```python
from build123d import *

# Parameters (mm, degrees)
SKETCH1_R           = 25
BOSS_EXTRUDE1_DEPTH = 2
SKETCH2_R           = 15
CUT_EXTRUDE1_DEPTH  = 5
CUT_EXTRUDE4_DEPTH  = 10
CIRPATTERN3_COUNT   = 20
CUT_EXTRUDE5_DEPTH  = 10
CIRPATTERN4_COUNT   = 10


with BuildPart() as part:
    # Sketch1 → Boss-Extrude1 (new body)
    with BuildSketch(Plane.XY):
        Circle(SKETCH1_R)
    extrude(amount=BOSS_EXTRUDE1_DEPTH)

    # Sketch2 → Cut-Extrude1 (cut)
    with BuildSketch(Plane(origin=(0, 0, 0), x_dir=(-1, 0, 0), z_dir=(0, 0, -1))):
        Circle(SKETCH2_R)
    extrude(amount=-CUT_EXTRUDE1_DEPTH, mode=Mode.SUBTRACT)

    # Sketch8 → Cut-Extrude4 (cut)
    with BuildSketch(Plane.XY.offset(2)):
        with BuildLine():
            Line((-1.502861851, 23.143578335), (-1.0312505, 16.38824879))
            Line((-1.0312505, 16.38824879), (1.0312505, 16.38824879))
            Line((1.0312505, 16.38824879), (1.478722794, 23.143578335))
            ThreePointArc((1.478722794, 23.143578335), (-0.012069528, 24.634370658), (-1.502861851, 23.143578335))
        make_face()
    cut_extrude4 = extrude(amount=-CUT_EXTRUDE4_DEPTH, mode=Mode.SUBTRACT)

    # CirPattern3: Cut-Extrude4 ×20 about axis
    cirpattern3_axis = Axis((0, 0, 0), (0, 0, 1))
    for i in range(1, CIRPATTERN3_COUNT):
        add(cut_extrude4.rotate(cirpattern3_axis, i * 360 / CIRPATTERN3_COUNT), mode=Mode.SUBTRACT)

    # Sketch9 → Cut-Extrude5 (cut)
    with BuildSketch(Plane.XY.offset(2)):
        with BuildLine():
            ThreePointArc((0, 16.155710659), (-2.535802961, 15.955459574), (-5.008743036, 15.359670572))
            ThreePointArc((-5.008743036, 15.359670572), (-5.251126101, 14.882712493), (-4.774168022, 14.640329428))
            ThreePointArc((-4.774168022, 14.640329428), (-2.417043421, 15.208215778), (0, 15.399088481))
            ThreePointArc((0, 15.399088481), (0.378311089, 15.77739957), (0, 16.155710659))
        make_face()
    cut_extrude5 = extrude(amount=-CUT_EXTRUDE5_DEPTH, mode=Mode.SUBTRACT)

    # CirPattern4: Cut-Extrude5 ×10 about axis
    cirpattern4_axis = Axis((0, 0, 0), (0, 0, 1))
    for i in range(1, CIRPATTERN4_COUNT):
        add(cut_extrude5.rotate(cirpattern4_axis, i * 360 / CIRPATTERN4_COUNT), mode=Mode.SUBTRACT)


solid = part.part
```
Input: part model. Units: mm. Frame: model coordinates. Give positions to 0.01 mm unless a question says otherwise; leave off trailing zeros. Loops run counter-clockwise (first coordinate to the right, second up) from the corner with the lowest first, then second, coordinate; pieces in that order, holes last. Notation, with made-up numbers: M 19,33 L 40,33 A21 ccw 40,71 Z; hole C 53,38 d6. An arc over 180 degrees is marked long. Answer as CSV lines item,"result". Start each with the question number.
1. Line query: L1, parallel to Y at x = 0, z = 0.8; L2, parallel to Y at x = -12, z = 0.8; L3, parallel to X at y = -4, z = 1.6. Output: solid intervals per line, ascending.
2. Section C-C on z = 1.3. State how many separate pieces and enclosed holes the cut face has, plus the area to 3 significant figures.
3. Pin query (flat end, axial travel): P1, Ø24, axis at x = 0, y = 0, coming from the -Z side. Return the tip coordinate at first contact, or that it passes through.
4. Section A-A on x = -7. Return loops of the section in (y, z), plus the area to 3 significant figures.
5. Section B-B on y = -19. Return loops of the section in (x, z).
Computed values:
1,L1,"y = -25 to -24.63, -16.39 to -16.16, -15.4 to -15, 15 to 15.4, 16.16 to 16.39, 24.63 to 25"
1,L2,"y = -21.93 to -18.99, -14.49 to -9, 9 to 9.65, 10.82 to 14.48, 18.95 to 21.93"
1,L3,"x = -24.68 to -14.46, 14.46 to 14.87, 15.65 to 24.68"
2,separate pieces,"1"
2,enclosed holes,"31"
2,area,"804 mm²"
3,P1,"passes through"
4,outline,"M -24,0 L -23.5,0 L -23.5,2 L -24,2 Z; M -17.66,0 L -14.56,0 L -14.56,2 L -17.66,2 Z; M -13.72,0 L -13.27,0 L -13.27,2 L -13.72,2 Z; M 13.27,0 L 17.63,0 L 17.63,2 L 13.27,2 Z; M 23.49,0 L 24,0 L 24,2 L 23.49,2 Z"
4,area,"17.8 mm²"
5,outline,"M -16.25,0 L -15.06,0 L -15.06,2 L -16.25,2 Z; M -12.01,0 L -7.54,0 L -7.54,2 L -12.01,2 Z; M -4.86,0 L -1.2,0 L -1.2,2 L -4.86,2 Z; M 1.21,0 L 4.87,0 L 4.87,2 L 1.21,2 Z; M 7.55,0 L 12.03,0 L 12.03,2 L 7.55,2 Z; M 15.08,0 L 16.25,0 L 16.25,2 L 15.08,2 Z"
